from build123d import *

# Parameters (mm, degrees)
SKETCH1_W           = 107.95
SKETCH1_H           = 236.535
SKETCH1_R           = 7.94
SKETCH1_R_2         = 2.86
SKETCH1_R_3         = 3.175
BOSS_EXTRUDE1_DEPTH = 3.175
FILLET1_R           = 25


with BuildPart() as part:
    # Sketch1 → Boss-Extrude1 (new body)
    with BuildSketch(Plane(origin=(0, 0, 0), x_dir=(0, 0, -1), z_dir=(1, 0, 0))):
        Rectangle(SKETCH1_W, SKETCH1_H)
        with Locations((0, -84.9275)):
            Circle(SKETCH1_R, mode=Mode.SUBTRACT)
        with Locations((20, -84.9275)):
            Circle(SKETCH1_R_2, mode=Mode.SUBTRACT)
        with Locations((-20, -84.9275)):
            Circle(SKETCH1_R_2, mode=Mode.SUBTRACT)
        with Locations((-34.925, 111.9175)):
            Circle(SKETCH1_R_3, mode=Mode.SUBTRACT)
        with Locations((34.925, 111.9175)):
            Circle(SKETCH1_R_3, mode=Mode.SUBTRACT)
    extrude(amount=BOSS_EXTRUDE1_DEPTH)

    # Fillet1
    fillet1_edges = [part.edges().sort_by_distance(p)[0] for p in [
        (1.5875, -118.2675, -53.975),
        (1.5875, -118.2675, 53.975),
    ]]
    fillet(fillet1_edges, radius=FILLET1_R)


solid = part.part
Geometry: final body of the model. Coordinates: model frame, mm. Round coordinates to 2 decimals unless told otherwise and drop trailing zeros. Loops run counter-clockwise (first coordinate to the right, second up) from the corner with the lowest first, then second, coordinate; pieces in that order, holes last. Notation, with made-up numbers: M -37.75,31.25 L 13.25,31.25 A5 ccw 13.25,39.25 Z; hole C 49.5,-6.75 d5. An arc over 180 degrees is marked long. One line per question, with ' | ' between items.
(1) Material intervals for line 1 along Y through (x, z) = (0.7, -20); line 2 along Y through (x, z) = (0.6, -19.5); line 3 along Y through (x, z) = (2.45, 49), sorted ascending. Write a range as from..to.
Check result:
line 1: y = -118.27..-87.79, -82.07..118.27 | line 2: y = -118.27..-87.74, -82.11..118.27 | line 3: y = -108.23..118.27
(2) Pull-direction query (Y, two-part tool) for faces 1 (the cylindrical face through (1.57, -82.09, -19.63)), 2 (the cylindrical face through (1.61, -110.75, 46.846)), 3 (the flat face through (0, 2, 1)), 4 (the cylindrical face through (1.57, -92.68, 1.72)); classes: +Y half, -Y half, draft (parallel to the pull), parting line (faces both ways), or undercut.
Check result:
face 1: undercut | face 2: -Y half | face 3: draft | face 4: undercut
(3) Cut plane A-A on z = 0. Return the cut outline in (x, y) (1 decimal).
Check result:
outline: M 0,-118.3 L 3.2,-118.3 L 3.2,-92.9 L 0,-92.9 Z; M 0,-77 L 3.2,-77 L 3.2,118.3 L 0,118.3 Z
(4) Contact query for a flat-ended pin moving along its axis: P1, Ø6.5, axis at y = -84.93, z = 20, coming from the +X side (3 decimals). Output: stop coordinate, or through.
Check result:
P1: stops at x = 3.175
(5) Cut plane C-C on x = 1.85. Give the number of separate pieces and of enclosed holes in the cut face, plus the area to 3 significant figures.
Check result:
separate pieces: 1 | enclosed holes: 5 | area: 25,000 mm2
(6) Cut plane B-B on z = -20. Return the cut outline in (x, y) (1 decimal), plus the area to 3 significant figures.
Check result:
outline: M 0,-118.3 L 3.2,-118.3 L 3.2,-87.8 L 0,-87.8 Z; M 0,-82.1 L 3.2,-82.1 L 3.2,118.3 L 0,118.3 Z | area: 733 mm2
